Autodesk Inventor part; units mm, degrees
ref_plane "YZ Plane" through (0, 0, 0) normal (1, 0, 0) x (0, 1, 0)
ref_plane "XZ Plane" through (0, 0, 0) normal (0, 1, 0) x (-1, 0, 0)
ref_plane "XY Plane" through (0, 0, 0) normal (0, 0, 1) x (1, 0, 0)
sketch "Esquisse1" plane through (0, 0, 0) normal (0, 0, 1) x (1, 0, 0)
  line L0 (0, 0) -> (0, 2)
  line L1 (0, 2) -> (15, 2)
  line L2 (15, 2) -> (10, 0)
  line L3 (10, 0) -> (0, 0)
  line L4 (0, 0) -> (3.6066, 0) construction
  dimension "d0" = 2
  dimension "d1" = 10
  dimension "d2" = 15
revolve "Révolution1" add sketch "Esquisse1" angle 360 about axis through (0, 0, 0) along (0, 1, 0)
sketch "Esquisse2" plane through (0, 0, 0) normal (0, -1, 0) x (1, 0, 0)
  circle A0 centre (0, 0) radius 9.9682
extrude "Extrusion1" add sketch "Esquisse2" along normal blind 2
sketch "Esquisse3" plane through (0, 0, 0) normal (1, 0, 0) x (0, 1, 0)
  line L0 (-2, 9.9682) -> (-2, -9.9682)
  line L1 (-2, 0) -> (-2, 9.9682)
  line L2 (-2, 9.9682) -> (-4, 15)
  line L3 (-4, 15) -> (-4, 0)
  line L4 (-4, 0) -> (-2, 0)
  point P0 (0, 0)
  dimension "d6" = 2
  dimension "d7" = 15
revolve "Révolution2" add sketch "Esquisse3" angle 360 about axis through (0, -4, 0) along (0, 1, 0)
sketch "Esquisse4" plane through (0, -4, 0) normal (0, -1, 0) x (1, 0, 0)
  circle A0 centre (0, 0) radius 2
  dimension "d9" = 4
extrude "Extrusion2" cut sketch "Esquisse4" against normal blind 6
properties part number "Hand polley" material "Plastique ABS"
Verification items for the finished model (mm, model axes). A direction names the side the tool comes from. Coordinates: 2 decimals unless noted, no trailing zeros. Write each loop counter-clockwise with the first axis right and the second up, starting at its lowest first coordinate (ties: lowest second). Pieces come first, ordered by that corner, then holes. Notation, with made-up numbers: (83.5, 37) -> (98.5, 37) arc R25 ccw to (98.5, 61) -> close; hole circle Ø7 at (50.5, 68.5). An arc over 180 degrees is marked (long way). One line per item, written item: value. Start each with the question number.
Q1. Thickness scan on L1, parallel to Z at x = 0, y = -0.75; L2, parallel to Y at x = 11.25, z = -2.5; L3, parallel to Y at x = -2.25, z = -13.5. Record the ranges inside material, lowest first. Write a range as from..to.
Q2. Cross-section at C-C on y = -1.5. Enter the section's corners in (x, z), and give its area (3 significant figures).
Q3. Mould release check, pull along X, two halves, no side actions. Record for faces 3 (the flat face through (-3, -4, 0)), 4 (the conical face through (9.837, 0.125, -3.098)), 5 (the cylindrical face through (0, -1, -2)): pulls with the +X half, pulls with the -X half, needs draft (parallel to the pull), parting line crosses it, or undercut.
Q4. Cross-section at D-D on y = 1.5. Enter the section's corners in (x, z), and give its area (3 significant figures).
Q5. Access from +Z, -Z, +X, -X, +Y, -Y to the whole of each face (thin tool, end or side, straight path). Record for faces 1 (the conical face through (10.038, -2.125, -2.229)), 2 (the flat face through (0, 2, 3)).
Checked values:
1. L1: z = -9.97..-2, 2..9.97
1. L2: y = -4..-2.62, 0.61..2
1. L3: y = -4..-3.48, 1.47..2
2. outline: circle Ø19.94 at (0, 0); hole circle Ø4 at (0, 0)
2. area: 300 mm²
3. face 3: needs draft
3. face 4: parting line crosses it
3. face 5: undercut
4. outline: circle Ø27.5 at (0, 0); hole circle Ø4 at (0, 0)
4. area: 581 mm²
5. face 1: none
5. face 2: +Z, -Z, +X, -X, +Y
